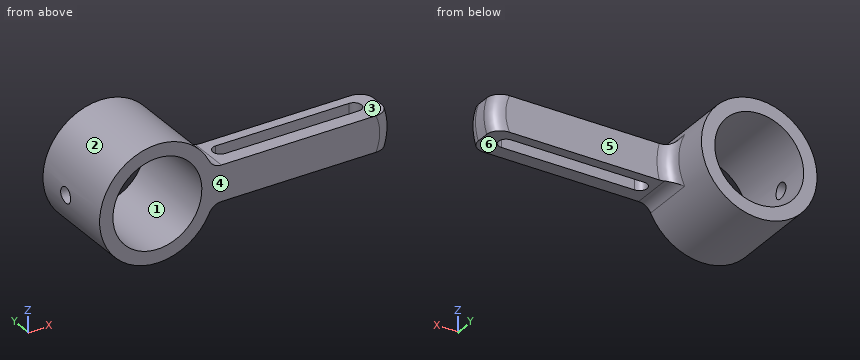
```python
from build123d import *

# Parameters (mm, degrees)
SKETCH_1_R          = 13
SKETCH_1_R_2        = 10
EXTRUDE_1_DEPTH     = 20
EXTRUDE_2_DEPTH     = 9
CUT_EXTRUDE_1_DEPTH = 60.14389233
FILLET_1_R          = 3
SKETCH_4_R          = 1.75
CUT_EXTRUDE_2_DEPTH = 59.120564438


# Read off the part's stored shape, not the designer's step: 凸台-拉伸2
with BuildPart() as part:
    # 草图1 → 凸台-拉伸1 (new body)
    with BuildSketch(Plane(origin=(0, 0, 0), x_dir=(1, 0, 0), z_dir=(0, 1, 0))):
        with Locations(Location((0, 0, 0), (0, 0, 270))):
            Circle(SKETCH_1_R)
        with Locations(Location((0, 0, 0), (0, 0, 270))):
            Circle(SKETCH_1_R_2, mode=Mode.SUBTRACT)
    extrude(amount=EXTRUDE_1_DEPTH)

    # 凸台-拉伸2 outline → 凸台-拉伸2 (add)
    with BuildSketch(Plane(origin=(0, 0, 0), x_dir=(1, 0, 0), z_dir=(0, 1, 0))):
        with BuildLine():
            ThreePointArc((52.369316877, -4), (53, 0), (52.369316877, 4))
            Line((52.369316877, 4), (12.369316877, 4))
            ThreePointArc((12.369316877, 4), (13, 0), (12.369316877, -4))
            Line((12.369316877, -4), (52.369316877, -4))
        make_face()
    extrude(amount=EXTRUDE_2_DEPTH)

    # 草图3 → 切除-拉伸1 (cut, through all)
    with BuildSketch(Plane.XY.offset(4)):
        with BuildLine():
            Line((17.369316877, 6.7), (47.369316877, 6.7))
            ThreePointArc((47.369316877, 6.7), (49.069316877, 5), (47.369316877, 3.3))
            Line((47.369316877, 3.3), (17.369316877, 3.3))
            ThreePointArc((17.369316877, 3.3), (15.669316877, 5), (17.369316877, 6.7))
        make_face()
    extrude(amount=-CUT_EXTRUDE_1_DEPTH, mode=Mode.SUBTRACT)

    # 圆角1
    fillet_1_edges = [part.edges().sort_by_distance(p)[0] for p in [
        (53, 9, 0),
        (53, 0, 0),
        (12.369316877, 4.5, -4),
        (13, 9, 0),
        (12.369316877, 4.5, 4),
    ]]
    fillet(fillet_1_edges, radius=FILLET_1_R)

    # 草图4 → 切除-拉伸2 (cut, through all)
    with BuildSketch(Plane(origin=(0, 0, 0), x_dir=(0, 0, -1), z_dir=(1, 0, 0))):
        with Locations((0, 12)):
            Circle(SKETCH_4_R)
    extrude(amount=-CUT_EXTRUDE_2_DEPTH, mode=Mode.SUBTRACT)


solid = part.part
```
Work out the finished part from the listing and answer in its coordinate system (mm). Face numbers are marked on the shaded views. A direction names the side the tool comes from. Give positions to 0.01 mm unless a question says otherwise; leave off trailing zeros. Write each loop counter-clockwise with the first axis right and the second up, starting at its lowest first coordinate (ties: lowest second). Pieces come first, ordered by that corner, then holes. Notation, with made-up numbers: (-31.5, -27) - (22.5, -27) arc R14 cw to (22.5, -9) - close; hole circle Ø9 at (8, -9). An arc over 180 degrees is marked (long way). Use one line per item in the form item = value.
1. A cutting plane is placed at B-B (x = 25). Write down the section's boundary in (y, z), and give its area (3 significant figures).
Filled in:
outline = (0, -4) - (3.3, -4) - (3.3, 4) - (0, 4) - close; (6.7, -4) - (9, -4) - (9, 4) - (6.7, 4) - close
area = 44.8 mm^2
2. A cutting plane is placed at A-A (y = 5). Write down the section's boundary in (x, z), and give its area (3 significant figures).
Filled in:
outline = (11.69, -5.69) arc R3 cw to (14.39, -4) - (15.67, -4) - (15.67, 4) - (14.39, 4) arc R3 cw to (11.69, 5.69) arc R13 ccw (long way) to start; (49.07, -4) - (52.37, -4) arc R13 ccw to (52.37, 4) - (49.07, 4) - close; hole circle Ø20 at (0, 0)
area = 271 mm^2
3. Determine the mould class of the marked faces 1, 2 and 3 for opening direction X: released by +X, released by -X, zero draft, split by the parting line, or undercut.
Filled in:
face_1 = undercut
face_2 = split by the parting line
face_3 = zero draft
4. A cutting plane is placed at C-C (z = 0). Write down the section's boundary in (x, y), and give its area (3 significant figures).
Filled in:
outline = (-13, 0) - (-10, 0) - (-10, 10.25) - (-13, 10.25) - close; (-13, 13.75) - (-10, 13.75) - (-10, 20) - (-13, 20) - close; (10, 0) - (50, 0) arc R3 ccw to (53, 3) - (53, 6) arc R3 ccw to (50, 9) - (16, 9) arc R3 cw to (13, 12) - (13, 20) - (10, 20) - close; hole (17.37, 3.3) - (47.37, 3.3) arc R1.7 ccw to (47.37, 6.7) - (17.37, 6.7) arc R1.7 ccw to start
area = 356 mm^2
5. Consider L1, parallel to Y at x = -11, z = 0; L2, parallel to Y at x = 28.5, z = 3.25; L3, parallel to X at y = 6.5, z = 0. Determine where each line is inside the solid, lowest interval first.
Filled in:
L1 = 0 to 10.25, 13.75 to 20
L2 = 0 to 3.3, 6.7 to 9
L3 = -13 to -10, 10 to 16.57, 48.17 to 52.96
6. A cutting plane is placed at D-D (y = 17.25). Write down the section's boundary in (x, z), and give its area (3 significant figures).
Filled in:
outline = circle Ø26 at (0, 0); hole circle Ø20 at (0, 0)
area = 217 mm^2
7. Each of these flat-tipped pins is pushed along its axis until it touches: pin 1 Ø12 at (x, z) = (33, -2.5) entering from +Y; pin 2 Ø3 at (y, z) = (12, 0) entering from +X; pin 3 Ø2 at (y, z) = (14, 8) entering from -X. Where does it stop, or does it pass through?
Filled in:
pin_1 = 9
pin_2 = 13.4
pin_3 = -10.95
8. For the marked faces 4, 5 and 6, determine the directions among +Z, -Z, +X, -X, +Y, -Y from which every point of the face is accessible in a straight line to the end or side of a thin tool.
Filled in:
face_4 = +Z, -Z, +X, -X, -Y
face_5 = +Z, -Z, +X, +Y
face_6 = -Z, +X, +Y, -Y
